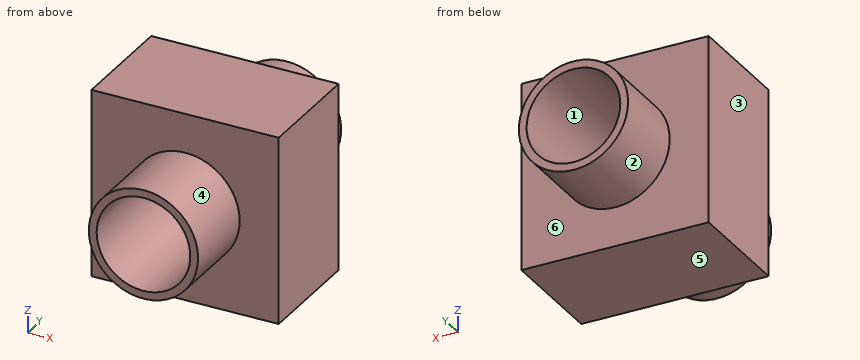
from build123d import *

# Parameters (mm, degrees)
F0_W     = 60
F0_H     = 60
F1_DEPTH = 36
F2_R     = 17.5
F3_DEPTH = 25
F4_R     = 17.5
F5_DEPTH = 25
F7_D     = 30


with BuildPart() as f1:
    # F0 (on Front) → F1 (new body)
    with BuildSketch(Plane.XZ):
        Rectangle(F0_W, F0_H)
    extrude(amount=-F1_DEPTH)

    # F2 (on face) → F3 (join)
    with BuildSketch(Plane.XZ):
        Circle(F2_R)
    extrude(amount=F3_DEPTH)

    # F4 (on face) → F5 (join)
    with BuildSketch(Plane(origin=(0, 36, 0), x_dir=(-1, 0, 0), z_dir=(0, 1, 0))):
        Circle(F4_R)
    extrude(amount=F5_DEPTH)

    # F7 (through all)
    with Locations(Plane.XZ.offset(25)):
        with Locations((0, 0)):
            Hole(F7_D / 2)


solid = f1.part
For this review, take the finished solid that the model builds, in its own axes (mm). Face numbers are marked on the shaded views. A direction names the side the tool comes from. Round coordinates to 2 decimals unless told otherwise and drop trailing zeros. Loops run counter-clockwise (first coordinate to the right, second up) from the corner with the lowest first, then second, coordinate; pieces in that order, holes last. Notation, with made-up numbers: (19.25, -0.5) - (48.25, -0.5) arc R29 ccw to (48.25, 23.5) - close; hole circle Ø3 at (59.25, -18.5). An arc over 180 degrees is marked (long way). Use one line per item in the form item = value.
1) We need section D-D on z = 26.5. Write out the cut boundary in (x, y), then the cut area to 3 significant figures.
Solutions:
outline = (-30, 0) - (30, 0) - (30, 36) - (-30, 36) - close
area = 2,160 mm2
2) We need section C-C on y = 29. Write out the cut boundary in (x, z), then the cut area to 3 significant figures.
Solutions:
outline = (-30, -30) - (30, -30) - (30, 30) - (-30, 30) - close; hole circle Ø30 at (0, 0)
area = 2,890 mm2
3) Mouldability with a two-part tool opening along Z and no side actions: class the marked faces 1, 2 and 3 as pulls with the +Z half, pulls with the -Z half, needs draft (parallel to the pull), parting line crosses it, or undercut.
Solutions:
face_1 = undercut
face_2 = parting line crosses it
face_3 = needs draft
4) Wall thickness on probe 1 along Z at (x, y) = (0, 14); probe 2 along Y at (x, z) = (-27, -9.5); probe 3 along Z at (x, y) = (0, 43): over which ranges is each line inside the solid? List them lowest first.
Solutions:
probe_1 = -30 to -15, 15 to 30
probe_2 = 0 to 36
probe_3 = -17.5 to -15, 15 to 17.5
5) We need section B-B on z = 0. Write out the cut boundary in (x, y), then the cut area to 3 significant figures.
Solutions:
outline = (-30, 0) - (-17.5, 0) - (-17.5, -25) - (-15, -25) - (-15, 61) - (-17.5, 61) - (-17.5, 36) - (-30, 36) - close; (15, -25) - (17.5, -25) - (17.5, 0) - (30, 0) - (30, 36) - (17.5, 36) - (17.5, 61) - (15, 61) - close
area = 1,330 mm2
6) Tool access review of the marked faces 4, 5 and 6: name each direction out of +Z, -Z, +X, -X, +Y, -Y from which nothing blocks a thin tool from reaching the whole face with its end or side.
Solutions:
face_4 = -Y
face_5 = -Z, +X, -X, +Y, -Y
face_6 = +Y
7) We need section A-A on x = 0. Write out the cut boundary in (y, z).
Solutions:
outline = (-25, -17.5) - (0, -17.5) - (0, -30) - (36, -30) - (36, -17.5) - (61, -17.5) - (61, -15) - (-25, -15) - close; (-25, 15) - (61, 15) - (61, 17.5) - (36, 17.5) - (36, 30) - (0, 30) - (0, 17.5) - (-25, 17.5) - close
8) Clearance check with a flat-ended pin moving along its axis: P1, Ø4, axis at x = 12, y = -4, coming from the -Z side. State where the tip first meets the part, or that it passes through.
Solutions:
P1 = -14.36
